Verification items for the finished model (mm, model axes). A direction names the side the tool comes from. Round coordinates to 2 decimals unless told otherwise and drop trailing zeros. Write each loop counter-clockwise with the first axis right and the second up, starting at its lowest first coordinate (ties: lowest second). Pieces come first, ordered by that corner, then holes. Notation, with made-up numbers: M 56.25,70.5 L 96.25,70.5 A18 ccw 96.25,96.5 Z; hole C 64,-36 d4. An arc over 180 degrees is marked long. Use a Markdown table: item, result. Add a question column.
from build123d import *

# Parameters (mm, degrees)
F0_W     = 50
F0_H     = 10
F1_DEPTH = 10
F2_SIZE  = 9.99999
F3_R     = 4
F4_DEPTH = 2


# Not quite as in the source:
# - a fillet or chamfer is up to 0.001 mm smaller than in the source, because OpenCascade refuses the exact size


with BuildPart() as f1:
    # F0 (on Top) → F1 (new body)
    with BuildSketch(Plane.XY):
        with Locations((-21.3684089482, 18.842792958)):
            Rectangle(F0_W, F0_H)
    extrude(amount=F1_DEPTH)

    # F2 (size 10 in the source; OpenCascade refuses exactly that, so slightly less here)
    f2_edges = [f1.edges().sort_by_distance(p)[0] for p in [
        (3.631591, 18.842793, 10),
    ]]
    chamfer(f2_edges, length=F2_SIZE)

    # F3 (on face) → F4 (join)
    with BuildSketch(Plane(origin=(1.8157955259, 0, 1.8157955259), x_dir=(0, 1, 0), z_dir=(0.7071067812, 0, 0.7071067812))):
        with Locations((18.842792958, 4.5031451526)):
            Circle(F3_R)
    extrude(amount=F4_DEPTH)


solid = f1.part
1. Scan lines: line 1 along X through (y, z) = (19.5, 9); line 2 along X through (y, z) = (22, 6.25); line 3 along X through (y, z) = (22.25, 4.5). Record each from-to range of solid material in increasing order. Write a range as from..to.
2. Cross-section at B-B on z = 1.75. Enter the section's corners in (x, y).
3. Access from +Z, -Z, +X, -X, +Y, -Y to the whole of each face (thin tool, end or side, straight path). Record for faces 4 (the flat face through (-1.44, 14.33, 5.07)), 5 (the flat face through (-27, 19, 10)).
4. Depth check by flat-ended pin: pin 1 Ø2 at (x, y) = (-2, 18) entering from +Z; pin 2 Ø1.5 at (y, z) = (21, 2.5) entering from +X; pin 3 Ø3 at (y, z) = (16.5, 3.5) entering from +X. Enter the tip coordinate at first touch or a pass-through.
5. Release check for a two-part mould opening along Z. For faces 1 (the flat face through (0.01, 18.79, 6.45)), 2 (the flat face through (-22, 13.843, 5)), 3 (the cylindrical face through (-0.796, 14.847, 5.822)) record: +Z half, -Z half, draft (parallel to the pull), parting line (faces both ways), or undercut.
Answer:
| question | item | result |
|---|---|---|
| 1 | line 1 | x = -46.37..-5.37, -2.95..-2.54 |
| 1 | line 2 | x = -46.37..0.21 |
| 1 | line 3 | x = -46.37..1.1 |
| 2 | outline | M -46.37,13.84 L 1.88,13.84 L 1.88,23.84 L -46.37,23.84 Z |
| 3 | face 4 | none |
| 3 | face 5 | +Z, +X, -X, +Y, -Y |
| 4 | pin 1 | stops at z = 9.24 |
| 4 | pin 2 | stops at x = 1.88 |
| 4 | pin 3 | stops at x = 2.81 |
| 5 | face 1 | +Z half |
| 5 | face 2 | draft |
| 5 | face 3 | undercut |
